Read the model definition and answer for the solid it produces. Units are mm, in the model's axes. Face numbers are marked on the shaded views. A direction names the side the tool comes from. Coordinates: 2 decimals unless noted, no trailing zeros. Write each loop counter-clockwise with the first axis right and the second up, starting at its lowest first coordinate (ties: lowest second). Pieces come first, ordered by that corner, then holes.
(1) Which of the six approach directions +Z, -Z, +X, -X, +Y, -Y give full straight-line access (tool end or side, diameter ignored) to the marked faces 5, 6 and 7?
(2) Determine the mould class of the marked faces 1, 2, 3 and 4 for opening direction Z: pulls with the +Z half, pulls with the -Z half, needs draft (parallel to the pull), parting line crosses it, or undercut.
(3) The part is cut by section A-A, the plane x = 9.6. Determine the outline of the cut face in (y, z).
(4) The part is cut by section B-B, the plane z = 26. Determine the outline of the cut face in (x, y), and give its area (3 significant figures).
(5) Given pin 1 (2 mm diameter, centred on y = -2, z = 7.5, fed in from +X); pin 2 (4 mm diameter, centred on x = 20.5, z = 17, fed in from +Y); pin 3 (5 mm diameter, centred on x = 11.5, y = -4.5, fed in from +Z); pin 4 (13 mm diameter, centred on x = 11.5, z = 16, fed in from -Y), each flat-ended and moving along its own axis, determine where each tip first touches the part or whether it passes through.
(6) The part is cut by section D-D, the plane y = -3.75. Determine the outline of the cut face in (x, z), and give its area (3 significant figures).
(7) The part is cut by section C-C, the plane z = 17. Determine the outline of the cut face in (x, y).
(8) Straight lines are drawn through the part: line 1 along Y through (x, z) = (9.6, 3.85); line 2 along X through (y, z) = (-9.75, 20.5); line 3 along Y through (x, z) = (8.25, 3). For each, find the intervals that lie inside material, in ascending order.
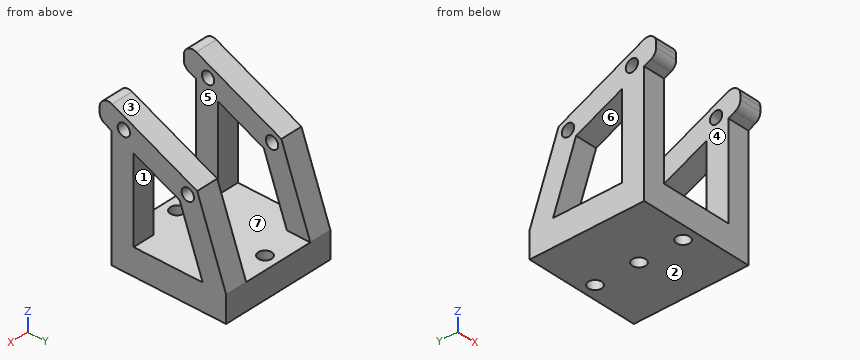
Autodesk Inventor part; units mm, degrees
ref_plane "YZ Plane" through (0, 0, 0) normal (1, 0, 0) x (0, 1, 0)
ref_plane "XZ Plane" through (0, 0, 0) normal (0, 1, 0) x (-1, 0, 0)
ref_plane "XY Plane" through (0, 0, 0) normal (0, 0, 1) x (1, 0, 0)
ref_plane "Arbeitsebene1" through (0, 0, 0) normal (0, 0, 1) x (1, 0, 0)
sketch "Skizze1" plane through (0, 0, 0) normal (0, 0, 1) x (1, 0, 0)
  circle A0 centre (19.6, 0) radius 1.5
  circle A1 centre (9.6, 0) radius 1.5
  circle A2 centre (-0.4, 0) radius 1.5
  circle A3 centre (9.6, -10) radius 1.5
  circle A4 centre (9.6, 10) radius 1.5
  arc A5 (22.5, -8.5328) -> (22.5, -11.4672) centre (19.6, -10) ccw
  arc A6 (22.5, 11.4672) -> (17.6036, 7.4354) centre (19.6, 10) ccw
  line L0 (-3.3, 16.2) -> (-22.5, 16.2)
  line L1 (-22.5, 16.2) -> (-22.5, -16.2)
  line L2 (-22.5, -16.2) -> (22.5, -16.2)
  line L3 (22.5, -16.2) -> (22.5, -11.4672)
  circle A7 centre (-0.4, -10) radius 3.25
  line L4 (-3.4, -13) -> (22.6, -13)
  line L5 (22.6, -13) -> (22.6, 13)
  line L6 (22.6, 13) -> (-3.4, 13)
  line L7 (-3.4, 13) -> (-3.4, -13)
  line L8 (-3.4, -13) -> (22.6, 13) construction
  line L9 (22.6, -13) -> (-3.4, 13) construction
  arc A8 (1.5964, 7.4354) -> (-2.3964, 7.4354) centre (-0.4, 10) ccw
  arc A9 (-2.3964, 7.4354) -> (1.5964, 7.4354) centre (-0.4, 4.8709) ccw
  arc A10 (-3.3, 23.4037) -> (-3.3, 26.3381) centre (-0.4, 24.8709) ccw
  line L10 (-3.3, 23.4037) -> (-3.3, 16.2)
  line L11 (22.5, -8.5328) -> (22.5, 3.4037)
  arc A11 (17.6036, 7.4354) -> (22.5, 3.4037) centre (19.6, 4.8709) ccw
  line L12 (22.5, 11.4672) -> (22.5, 23.4037)
  arc A12 (22.5, 26.3381) -> (22.5, 23.4037) centre (19.6, 24.8709) ccw
  line L13 (22.5, 26.3381) -> (22.5, 28.2)
  line L14 (22.5, 28.2) -> (-3.3, 28.2)
  line L15 (-3.3, 28.2) -> (-3.3, 26.3381)
  point P0 (0, 0)
  point P1 (22.5, 16.2)
  dimension "d0" = 26
  dimension "d1" = 26
extrude "Extrusion1" add sketch "Skizze1" along normal blind 6 contours L11 A11 A6 L6 L12 L5 L4 L3 A5 | A5 L4 A7 L7 A9 A8 L6 A6 A11 L11 | A5 L3 L4 | L4 A7 L7 | L4 L7 A7 | L6 L12 A6 | A8 A9 L7 L6 | A8 L7 L6 | L7 A8 A9
sketch "Skizze2" plane through (-3.4, -13, 0) normal (-1, 0, 0) x (0, 0, 1)
  line L0 (0, 26) -> (0, 0)
  line L1 (0, 0) -> (6, 0)
  line L2 (6, 26) -> (6, 0)
  line L3 (0, 26) -> (6, 26)
  line L4 (6, 26) -> (23.9972, 19.4291)
  line L5 (23.9972, 19.4291) -> (32.8468, 0)
  line L6 (32.8468, 0) -> (27.3526, 0)
  line L7 (6, 24.5) -> (6, 20.6772)
  line L8 (27.3526, 0) -> (6, 0)
  line L9 (6, 20.6772) -> (20.3151, 15.4507)
  line L10 (20.3151, 15.4507) -> (25.0752, 5)
  line L11 (25.0752, 5) -> (6, 5)
  line L12 (32.8468, 0) -> (32.7967, 0.1099)
  line L13 (30.9766, -2.7191) -> (29.8778, -2.7191)
  line L14 (28.0577, -1.5481) -> (27.3526, 0)
  arc A0 (30.9766, -2.7191) -> (32.7967, 0.1099) centre (30.9766, -0.7191) ccw
  arc A1 (28.0577, -1.5481) -> (29.8778, -2.7191) centre (29.8778, -0.7191) ccw
  circle A2 centre (28.7957, 2.7835) radius 1.4
  circle A3 centre (22.3001, 17.2899) radius 1.4
  point P0 (0, 13)
  point P1 (32.8429, 0)
  point P2 (32.7967, 0.1099)
  dimension "d4" = 5
  dimension "d6" = 5
  dimension "d7" = 5
  dimension "d8" = 0
  dimension "d9" = 2
  dimension "d12" = 2.8
  dimension "d13" = 2.8
extrude "Extrusion2" add sketch "Skizze2" against normal blind 5 contours L3 L2 L1 L0 | L4 L5 A0 L6 L8 L2 L11 L10 L9 | L6 A0 L13 A1 L14
ref_plane "Arbeitsebene2" through (9.6, -13, 0) normal (-1, 0, 0) x (0, 0, 1)
mirror "Spiegeln1" about plane through (9.6, -13, 0) normal (-1, 0, 0) of "Extrusion2"
properties part number "Gripper_linear_finger"
Computed:
1. face 5: +Z, +Y, -Y
1. face 6: +X, -X
1. face 7: none
2. face 1: undercut
2. face 2: pulls with the -Z half
2. face 3: pulls with the +Z half
2. face 4: needs draft
3. outline: (-13, 0) - (-11.5, 0) - (-11.5, 6) - (-13, 6) - close; (-8.5, 0) - (-1.5, 0) - (-1.5, 6) - (-8.5, 6) - close; (1.5, 0) - (8.5, 0) - (8.5, 6) - (1.5, 6) - close; (11.5, 0) - (13, 0) - (13, 6) - (11.5, 6) - close
4. outline: (-3.4, -13) - (1.6, -13) - (1.6, 2.03) - (-3.4, 2.03) - close; (17.6, -13) - (22.6, -13) - (22.6, 2.03) - (17.6, 2.03) - close
4. area: 150 mm2
5. pin 1: passes through
5. pin 2: stops at y = 9.71
5. pin 3: stops at z = 6
5. pin 4: stops at y = -13
6. outline: (-3.4, 0) - (22.6, 0) - (22.6, 6) - (-3.4, 6) - close; (-3.4, 23.14) - (1.6, 23.14) - (1.6, 28.63) - (-3.4, 28.63) - close; (17.6, 23.14) - (22.6, 23.14) - (22.6, 28.63) - (17.6, 28.63) - close
6. area: 211 mm2
7. outline: (-3.4, -13) - (1.6, -13) - (1.6, -8) - (-3.4, -8) - close; (-3.4, 3.66) - (1.6, 3.66) - (1.6, 8.98) - (-3.4, 8.98) - close; (17.6, -13) - (22.6, -13) - (22.6, -8) - (17.6, -8) - close; (17.6, 3.66) - (22.6, 3.66) - (22.6, 8.98) - (17.6, 8.98) - close
8. line 1: y = -13 to -11.5, -8.5 to -1.5, 1.5 to 8.5, 11.5 to 13
8. line 2: x = -3.4 to 1.6, 17.6 to 22.6
8. line 3: y = -13 to -10.65, -9.35 to -0.65, 0.65 to 9.35, 10.65 to 13
